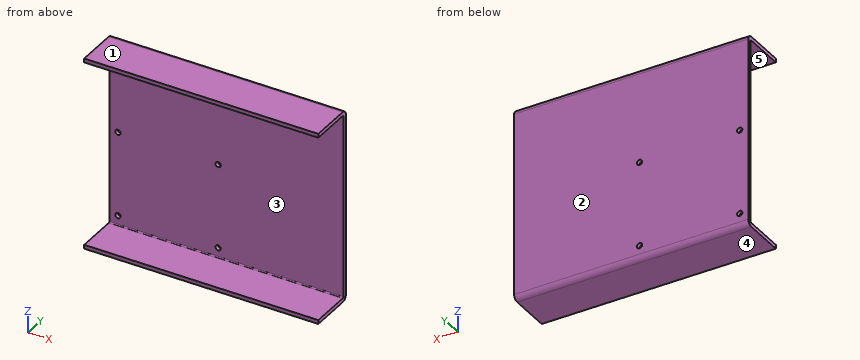
```python
from build123d import *

# Parameters (mm, degrees)
SKETCH2_W                      = 190
SKETCH2_H                      = 150
BASE_FLANGE1_DEPTH             = 3.175
EDGE_FLANGE1_STRIP_W           = 14.578
EDGE_FLANGE1_STRIP_H           = 3.175
EDGE_FLANGE1_STRIP_CUT_DEPTH   = 190
EDGE_FLANGE1_STRIP_2_W         = 14.578
EDGE_FLANGE1_STRIP_2_H         = 3.175
EDGE_FLANGE1_STRIP_CUT_2_DEPTH = 190
EDGE_FLANGE1_DEPTH             = 190
EDGE_FLANGE1_BEND_DEPTH        = 190
F_6_CLEARANCE_HOLE1_D          = 4.3053
F_6_CLEARANCE_HOLE1_DEPTH      = 17.23
F_6_CLEARANCE_HOLE1_TIP        = 1.293442612


# Sheet-metal steps are written as plain solids
with BuildPart() as part:
    # Sketch2 → Base-Flange1 (new body)
    with BuildSketch(Plane(origin=(0, 0, 0), x_dir=(1, 0, 0), z_dir=(0, 1, 0))):
        Rectangle(SKETCH2_W, SKETCH2_H)
    extrude(amount=-BASE_FLANGE1_DEPTH)

    # Edge-Flange1 strip (across the edge) → Edge-Flange1 strip cut (cut)
    with BuildSketch(Plane(origin=(95, -3.175, 75.1), x_dir=(0, 0, -1), z_dir=(-1, 0, 0))):
        with Locations((-6.4, -1.5875)):
            Rectangle(EDGE_FLANGE1_STRIP_W, EDGE_FLANGE1_STRIP_H)
    extrude(amount=EDGE_FLANGE1_STRIP_CUT_DEPTH, mode=Mode.SUBTRACT)

    # Edge-Flange1 strip 2 (across the edge) → Edge-Flange1 strip cut 2 (cut)
    with BuildSketch(Plane(origin=(-95, -3.175, -75.1), x_dir=(0, 0, 1), z_dir=(1, 0, 0))):
        with Locations((-6.4, -1.5875)):
            Rectangle(EDGE_FLANGE1_STRIP_2_W, EDGE_FLANGE1_STRIP_2_H)
    extrude(amount=EDGE_FLANGE1_STRIP_CUT_2_DEPTH, mode=Mode.SUBTRACT)

    # Edge-Flange1 section (across the edge) → Edge-Flange1 (add)
    with BuildSketch(Plane(origin=(95, -3.175, 75.1), x_dir=(0, 0, -1), z_dir=(-1, 0, 0))):
        with BuildLine():
            Line((-3.175, 0.889), (-3.175, 34))
            Line((-3.175, 34), (0, 34))
            Line((0, 34), (0, 0.889))
            ThreePointArc((0, 0.889), (0.260382072, 0.260382072), (0.889, 0))
            Line((0.889, 0), (0.889, -3.175))
            ThreePointArc((0.889, -3.175), (-1.984681959, -1.984681959), (-3.175, 0.889))
        make_face()
    extrude(amount=EDGE_FLANGE1_DEPTH)

    # Edge-Flange1 section 2 (across the edge) → Edge-Flange1 bend (add)
    with BuildSketch(Plane(origin=(-95, -3.175, -75.1), x_dir=(0, 0, 1), z_dir=(1, 0, 0))):
        with BuildLine():
            Line((-3.175, 0.889), (-3.175, 34))
            Line((-3.175, 34), (0, 34))
            Line((0, 34), (0, 0.889))
            ThreePointArc((0, 0.889), (0.260382072, 0.260382072), (0.889, 0))
            Line((0.889, 0), (0.889, -3.175))
            ThreePointArc((0.889, -3.175), (-1.984681959, -1.984681959), (-3.175, 0.889))
        make_face()
    extrude(amount=EDGE_FLANGE1_BEND_DEPTH)

    # #6 Clearance Hole1
    with Locations(Plane(origin=(0, 0, 0), x_dir=(1, 0, 0), z_dir=(0, 1, 0))):
        with Locations((-88.015, 67.226), (-6.735, 67.226), (-6.735, -1.354), (-88.015, -1.354)):
            Hole(F_6_CLEARANCE_HOLE1_D / 2, depth=F_6_CLEARANCE_HOLE1_DEPTH)
            with Locations((0, 0, -(F_6_CLEARANCE_HOLE1_DEPTH + F_6_CLEARANCE_HOLE1_TIP / 2))):  # 118° drill point
                Cone(0, F_6_CLEARANCE_HOLE1_D / 2, F_6_CLEARANCE_HOLE1_TIP, mode=Mode.SUBTRACT)


solid = part.part
```
Read the model definition and answer for the solid it produces. Units are mm, in the model's axes. Face numbers are marked on the shaded views. A direction names the side the tool comes from. Give positions to 0.01 mm unless a question says otherwise; leave off trailing zeros. Write each loop counter-clockwise with the first axis right and the second up, starting at its lowest first coordinate (ties: lowest second). Pieces come first, ordered by that corner, then holes. Notation, with made-up numbers: (66, 26.5) -> (97, 26.5) arc R27 ccw to (97, 51.5) -> close; hole circle Ø5 at (58, 24.25). An arc over 180 degrees is marked (long way). Answer as a JSON object with one key per item and string values.
1) Straight lines are drawn through the part: probe 1 along Z at (x, y) = (3, -13) (3 decimals); probe 2 along Y at (x, z) = (-28, 27.5) (3 decimals); probe 3 along Z at (x, y) = (47, -2). For each, find the intervals that lie inside material, in ascending order. Write a range as from..to.
Findings below:
{"probe 1": "z = -78.275..-75.1, 75.1..78.275", "probe 2": "y = -3.175..0", "probe 3": "z = -77.71..77.71"}
2) A tool of negligible diameter and unlimited length cuts with its end or side. For the marked faces 4 and 5, from which of +Z, -Z, +X, -X, +Y, -Y can it reach the whole face along a straight path? Write none if from no direction.
Findings below:
{"face 4": "-Z, +X, -X, +Y, -Y", "face 5": "+X, -X, -Y"}
3) Section C-C on z = -22 is taken. Write down the section's boundary in (x, y) (3 decimals).
Findings below:
{"outline": "(-95, -3.175) -> (95, -3.175) -> (95, 0) -> (-95, 0) -> close"}
4) A flat-ended cylindrical pin translates along its axis: pin 1 Ø5 at (x, z) = (-88.015, 1.354) entering from -Y (3 decimals). Find the tip coordinate at first contact, or state that the pin passes through.
Findings below:
{"pin 1": "stops at y = -3.175"}
5) Section B-B on x = 60.5 is taken. Write down the section's boundary in (y, z) (3 decimals).
Findings below:
{"outline": "(-37.175, -78.275) -> (-4.064, -78.275) arc R4.064 ccw to (0, -74.211) -> (0, 74.211) arc R4.064 ccw to (-4.064, 78.275) -> (-37.175, 78.275) -> (-37.175, 75.1) -> (-4.064, 75.1) arc R0.889 cw to (-3.175, 74.211) -> (-3.175, -74.211) arc R0.889 cw to (-4.064, -75.1) -> (-37.175, -75.1) -> close"}
6) For a pull along Z with two mould halves and no side action, classify the marked faces 1, 2 and 3 as pulls with the +Z half, pulls with the -Z half, needs draft (parallel to the pull), parting line crosses it, or undercut.
Findings below:
{"face 1": "pulls with the +Z half", "face 2": "needs draft", "face 3": "undercut"}
7) Section A-A on y = -18.5 is taken. Write down the section's boundary in (x, z) (3 decimals), then the cut area to 3 significant figures.
Findings below:
{"outline": "(-95, -78.275) -> (95, -78.275) -> (95, -75.1) -> (-95, -75.1) -> close; (-95, 75.1) -> (95, 75.1) -> (95, 78.275) -> (-95, 78.275) -> close", "area": "1,210 mm^2"}
